```python
from build123d import *

# Parameters (mm, degrees)
SKETCH_1_R          = 10
SKETCH_1_R_2        = 2.5
EXTRUDE_1_DEPTH     = 70
SKETCH_2_W          = 60
SKETCH_2_H          = 40
SKETCH_2_H_2        = 50
CUT_EXTRUDE_1_DEPTH = 70
CUT_EXTRUDE_2_DEPTH = 60


with BuildPart() as part:
    # 草图1 → 凸台-拉伸1 (new body)
    with BuildSketch(Plane.XY):
        with BuildLine():
            Line((-15, 90), (-15, 0))
            ThreePointArc((-15, 0), (0, -15), (15, 0))
            Line((15, 0), (15, 90))
            ThreePointArc((15, 90), (0, 105), (-15, 90))
        make_face()
        Circle(SKETCH_1_R, mode=Mode.SUBTRACT)
        with Locations((0, 90)):
            Circle(SKETCH_1_R_2, mode=Mode.SUBTRACT)
    extrude(amount=EXTRUDE_1_DEPTH)

    # 草图2 → 切除-拉伸1 (cut)
    with BuildSketch(Plane.ZY.offset(15)):
        with Locations((35, 0)):
            Rectangle(SKETCH_2_W, SKETCH_2_H)
        with Locations((35, 95)):
            Rectangle(SKETCH_2_W, SKETCH_2_H_2)
    extrude(amount=-CUT_EXTRUDE_1_DEPTH, mode=Mode.SUBTRACT)

    # 草图3 → 切除-拉伸2 (cut)
    with BuildSketch(Plane(origin=(0, 0, 65), x_dir=(-1, 0, 0), z_dir=(0, 0, -1))):
        with BuildLine():
            Line((15, 55), (15, 70))
            Line((15, 70), (1.38e-07, 70))
            ThreePointArc((1.38e-07, 70), (10.606601767, 65.606601669), (15, 55))
        make_face()
        with BuildLine():
            ThreePointArc((-15, 55), (-10.606601669, 65.606601767), (1.38e-07, 70))
            Line((1.38e-07, 70), (-15, 70))
            Line((-15, 70), (-15, 55))
        make_face()
        with BuildLine():
            ThreePointArc((0, 20), (-10.606601718, 24.393398282), (-15, 35))
            Line((-15, 35), (-15, 20))
            Line((-15, 20), (0, 20))
        make_face()
        with BuildLine():
            ThreePointArc((15, 35), (10.606601718, 24.393398282), (0, 20))
            Line((0, 20), (15, 20))
            Line((15, 20), (15, 35))
        make_face()
    extrude(amount=CUT_EXTRUDE_2_DEPTH, mode=Mode.SUBTRACT)


solid = part.part
```
Geometry check sheet. Reference: the model listing, model coordinates, mm. Coordinates: 2 decimals unless noted, no trailing zeros. Loops run counter-clockwise (first coordinate to the right, second up) from the corner with the lowest first, then second, coordinate; pieces in that order, holes last.
Item 1: Thickness scan on line 1 (Y direction, x = 0, z = 3.7); line 2 (Z direction, x = -9, y = 18); line 3 (X direction, y = 90, z = 67.8). Record the ranges inside material, lowest first.
Item 2: Go/stop test with flat-tipped pins: pin 1 Ø15 at (x, y) = (4.5, 74) entering from -Z; pin 2 Ø3 at (x, z) = (6, 12.5) entering from +Y; pin 3 Ø1.5 at (x, z) = (8.5, 36) entering from +Y. Record where each tip stops, or that it passes through.
Item 3: Sectioned sample at A-A, the plane y = 13.5. Record the boundary of the cut face in (x, z), then the cut area to 3 significant figures.
Item 4: Sectioned sample at B-B, the plane x = 5. Record the boundary of the cut face in (y, z), then the cut area to 3 significant figures.
Item 5: Sectioned sample at C-C, the plane z = 12. Record the boundary of the cut face in (x, y).
Item 6: Sectioned sample at D-D, the plane x = -7.5. Record the boundary of the cut face in (y, z), then the cut area to 3 significant figures.
Item 7: Release check for a two-part mould opening along X. For faces 1 (the face through (0, 105, 2)), 2 (the face through (-0.33, 92.48, 2.46)), 3 (the face through (-15, 46, 35)), 4 (the face through (-2.17, -9.76, 2.46)) record: released by +X, released by -X, zero draft, split by the parting line, or undercut.
Check result:
1. line 1: y = -15 to -10, 10 to 87.5, 92.5 to 105
1. line 2: z = 0 to 5, 65 to 70
1. line 3: x = -15 to -2.5, 2.5 to 15
2. pin 1: stops at z = 0
2. pin 2: stops at y = 69.31
2. pin 3: stops at y = 67.84
3. outline: (-15, 0) - (15, 0) - (15, 5) - (-15, 5) - close; (-15, 65) - (15, 65) - (15, 70) - (-15, 70) - close
3. area: 300 mm2
4. outline: (-14.14, 0) - (-8.66, 0) - (-8.66, 5) - (-14.14, 5) - close; (-14.14, 65) - (-8.66, 65) - (-8.66, 70) - (-14.14, 70) - close; (8.66, 0) - (104.14, 0) - (104.14, 5) - (69.14, 5) - (69.14, 65) - (104.14, 65) - (104.14, 70) - (8.66, 70) - (8.66, 65) - (20.86, 65) - (20.86, 5) - (8.66, 5) - close
4. area: 3,910 mm2
5. outline: (-15, 35) arc R15 ccw to (15, 35) - (15, 55) arc R15 ccw to (-15, 55) - close
6. outline: (-12.99, 0) - (-6.61, 0) - (-6.61, 5) - (-12.99, 5) - close; (-12.99, 65) - (-6.61, 65) - (-6.61, 70) - (-12.99, 70) - close; (6.61, 0) - (102.99, 0) - (102.99, 5) - (67.99, 5) - (67.99, 65) - (102.99, 65) - (102.99, 70) - (6.61, 70) - (6.61, 65) - (22.01, 65) - (22.01, 5) - (6.61, 5) - close
6. area: 3,790 mm2
7. face 1: split by the parting line
7. face 2: undercut
7. face 3: released by -X
7. face 4: undercut
